Input: part model. Units: mm. Frame: model coordinates. Face numbers are marked on the shaded views. A direction names the side the tool comes from. Round coordinates to 2 decimals unless told otherwise and drop trailing zeros. Loops run counter-clockwise (first coordinate to the right, second up) from the corner with the lowest first, then second, coordinate; pieces in that order, holes last. Notation, with made-up numbers: M 73,89 L 108,89 A18 cw 108,106 Z; hole C -2,-34 d10. An arc over 180 degrees is marked long. Return JSON: item names as keys, results as strings. Group by question number.
1) Mould query, pull axis Y, two halves, no side actions, for the marked faces 4, 5, 6 and 7. Classes: +Y half, -Y half, draft (parallel to the pull), parting line (faces both ways), or undercut.
2) Section C-C (y = 82.55). Output: boundary loops of the cut face in (x, z) (3 decimals).
3) Material intervals for line 1 (X direction, y = 82.55, z = -115); line 2 (Y direction, x = 38.1, z = -127) (3 decimals); line 3 (Z direction, x = 6, y = 52) (3 decimals), sorted ascending. Write a range as from..to.
4) Contact query for flat-ended pins moving along their axis: P1, Ø1, axis at x = -4.5, z = -40, coming from the +Y side; P2, Ø23, axis at x = 78, z = -17.5, coming from the +Y side (3 decimals); P3, Ø1, axis at x = 51.5, y = -1.5, coming from the +Z side (3 decimals). Output: stop coordinate, or through.
5) Access query for the marked faces 1, 2 and 3. Directions: +Z, -Z, +X, -X, +Y, -Y. A direction counts if a zero-diameter tool reaches every point of the face in a straight line with its end or side. Return the directions, or none.
6) Section D-D (z = -14.5). Output: boundary loops of the cut face in (x, y) (3 decimals).
7) Section B-B (z = -110). Output: boundary loops of the cut face in (x, y) (3 decimals), plus the area to 3 significant figures.
8) Section A-A (x = 38.1). Output: boundary loops of the cut face in (y, z) (3 decimals).
Autodesk Inventor part; units mm, degrees
ref_plane "YZ Plane" through (0, 0, 0) normal (1, 0, 0) x (0, 1, 0)
ref_plane "XZ Plane" through (0, 0, 0) normal (0, 1, 0) x (-1, 0, 0)
ref_plane "XY Plane" through (0, 0, 0) normal (0, 0, 1) x (1, 0, 0)
sketch "Sketch1" plane through (0, 0, 0) normal (0, 0, 1) x (1, 0, 0)
  line L0 (0, 0) -> (76.2, 0)
  line L1 (76.2, 0) -> (76.2, -3.175)
  line L2 (76.2, -3.175) -> (101.6, -3.175)
  line L3 (101.6, -3.175) -> (101.6, 41.275)
  line L4 (101.6, 41.275) -> (69.85, 41.275)
  line L5 (69.85, 41.275) -> (69.85, 31.75)
  line L6 (69.85, 31.75) -> (6.35, 31.75)
  line L7 (6.35, 31.75) -> (6.35, 41.275)
  line L8 (6.35, 41.275) -> (-25.4, 41.275)
  line L9 (-25.4, 41.275) -> (-25.4, -3.175)
  line L10 (-25.4, -3.175) -> (0, -3.175)
  line L11 (0, -3.175) -> (0, 0)
  dimension "d0" = 76.2
  dimension "d2" = 25.4
  dimension "d3" = 44.45
  dimension "d4" = 31.75
  dimension "d5" = 9.525
  dimension "d6" = 63.5
  dimension "d8" = 9.525
  dimension "d9" = 31.75
  dimension "d18" = 25.4
extrude "Extrusion3" add sketch "Sketch1" against normal blind 136.525
sketch "Sketch5" plane through (101.6, -3.175, 0) normal (1, 0, 0) x (0, 0, -1)
  line L0 (0, 44.45) -> (0, 0)
  line L1 (0, 44.45) -> (136.525, 44.45)
  line L2 (28.575, 44.45) -> (28.575, 34.925)
  line L3 (136.525, 0) -> (136.525, 44.45)
  line L4 (136.525, 44.45) -> (28.575, 44.45)
  line L5 (0, 34.925) -> (136.525, 34.925)
  line L6 (28.575, 34.925) -> (136.525, 34.925)
  line L7 (136.525, 34.925) -> (136.525, 44.45)
  point P0 (0, 3.175)
  dimension "d21" = 28.575
  dimension "d22" = 9.525
extrude "Extrusion4" cut sketch "Sketch5" against normal through all contours L1 L3 L5 L2
sketch "Sketch6" plane through (101.6, -3.175, 0) normal (1, 0, 0) x (0, 0, -1)
  line L0 (136.525, 0) -> (136.525, 136.525)
  line L1 (136.525, 136.525) -> (104.775, 136.525)
  line L2 (104.775, 136.525) -> (104.775, 0)
  line L3 (0, 0) -> (136.525, 0)
  point P0 (0, 3.175)
  dimension "d25" = 136.525
  dimension "d26" = 31.75
extrude "Extrusion5" add sketch "Sketch6" against normal blind 127
sketch "Sketch7" plane through (101.6, -3.175, 0) normal (1, 0, 0) x (0, 0, -1)
  line L0 (28.575, 34.925) -> (28.575, 44.45)
  line L1 (28.575, 44.45) -> (28.575, 34.925)
  line L2 (28.575, 34.925) -> (92.075, 34.925)
  line L3 (104.775, 136.525) -> (136.525, 136.525)
  line L4 (104.775, 47.625) -> (104.775, 136.525)
  line L5 (104.775, 136.525) -> (136.525, 136.525)
  line L6 (136.525, 136.525) -> (136.525, 0)
  line L7 (136.525, 0) -> (0, 0)
  line L8 (0, 0) -> (0, 44.45)
  line L9 (0, 44.45) -> (28.575, 44.45)
  arc A0 (92.075, 34.925) -> (104.775, 47.625) centre (92.075, 47.625) ccw
  line L10 (28.575, 34.925) -> (28.575, 0)
  line L11 (0, 0) -> (104.775, 0)
  point P0 (0, 3.175)
  point P1 (104.775, 34.925)
  point P2 (28.575, 0)
  dimension "d29" = 12.7
extrude "Extrusion6" add sketch "Sketch7" against normal blind 127 contours L2 A0 L4 L3 L6 L7 L10
sketch "Sketch8" plane through (-25.4, 133.35, -104.775) normal (0, 0, 1) x (1, 0, 0)
  line L0 (114.3, 0) -> (12.7, 0)
  line L1 (0, -12.7) -> (0, -88.9)
  line L2 (127, 0) -> (127, -136.525)
  arc A0 (127, -12.7) -> (114.3, 0) centre (114.3, -12.7) ccw
  arc A1 (12.7, 0) -> (0, -12.7) centre (12.7, -12.7) ccw
  line L3 (0, -88.9) -> (0, 0)
  line L4 (127, 0) -> (0, 0)
  line L5 (114.3, 0) -> (127, 0)
  line L6 (127, 0) -> (127, -12.7)
  point P0 (25.4, -133.35)
  point P1 (127, -12.7)
  dimension "d32" = 12.7
  dimension "d33" = 12.7
extrude "Extrusion7" cut sketch "Sketch8" against normal through all contours L4 L2 A0
sketch "Sketch9" plane through (-25.4, 44.45, -104.775) normal (0, 0, 1) x (1, 0, 0)
  line L0 (114.3, 88.9) -> (0, 88.9)
  line L1 (12.7, 88.9) -> (69.85, 88.9)
  line L2 (0, 76.2) -> (0, 46.0375)
  line L3 (0, 0) -> (0, 88.9)
  arc A0 (12.7, 88.9) -> (0, 76.2) centre (12.7, 76.2) ccw
  line L4 (0, 76.2) -> (0, 88.9)
  point P0 (25.4, -44.45)
  dimension "d36" = 12.7
extrude "Extrusion8" cut sketch "Sketch9" against normal through all
sketch "Sketch10" plane through (-25.4, 44.45, -104.775) normal (0, 0, 1) x (1, 0, 0)
  line L0 (127, 76.2) -> (127, 0)
  line L1 (114.3, 88.9) -> (12.7, 88.9)
  point P0 (25.4, -44.45)
  point P1 (63.5, 38.1)
  point P2 (63.5, 38.1)
  dimension "d39" = 63.5
  dimension "d40" = 50.8
hole "Hole1" at (38.1, 82.55, -104.775) at (38.1, 82.55, -104.775) direction (0, 0, -1) diameter 50.8 end through all
properties part number "Assignment 2.2 - Tube Mount"
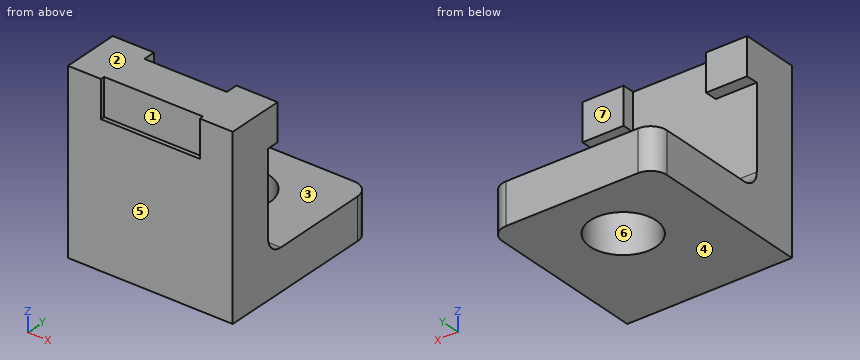
Returned:
{
 "1": {"face 4": "draft", "face 5": "-Y half", "face 6": "undercut", "face 7": "+Y half"},
 "2": {"outline": "M -25.4,-136.525 L 12.7,-136.525 L 12.7,-104.775 L -25.4,-104.775 Z; M 63.5,-136.525 L 101.6,-136.525 L 101.6,-104.775 L 63.5,-104.775 Z"},
 "3": {"line 1": "x = -25.4..12.7, 63.5..101.6", "line 2": "y = -3.175..57.15, 107.95..133.35", "line 3": "z = -136.525..-104.775"},
 "4": {"P1": "stops at y = 31.75", "P2": "stops at y = 41.275", "P3": "stops at z = -28.575"},
 "5": {"face 1": "+Z, -Y", "face 2": "+Z, +X, -X, +Y, -Y", "face 3": "+Z, +X, -X, +Y"},
 "6": {"outline": "M -25.4,-3.175 L 0,-3.175 L 0,0 L 76.2,0 L 76.2,-3.175 L 101.6,-3.175 L 101.6,41.275 L 69.85,41.275 L 69.85,31.75 L 6.35,31.75 L 6.35,41.275 L -25.4,41.275 Z"},
 "7": {"outline": "M -25.4,-3.175 L 101.6,-3.175 L 101.6,120.65 A12.7 ccw 88.9,133.35 L -12.7,133.35 A12.7 ccw -25.4,120.65 Z; hole C 38.1,82.55 d50.8", "area": "15,200 mm^2"},
 "8": {"outline": "M -3.175,-136.525 L 57.15,-136.525 L 57.15,-104.775 L 44.45,-104.775 A12.7 cw 31.75,-92.075 L 31.75,0 L 0,0 L 0,-28.575 L -3.175,-28.575 Z; M 107.95,-136.525 L 133.35,-136.525 L 133.35,-104.775 L 107.95,-104.775 Z"}
}
